The model under review builds one solid part; all positions refer to its coordinate system, in mm. Face numbers are marked on the shaded views. A direction names the side the tool comes from. Round coordinates to 2 decimals unless told otherwise and drop trailing zeros. Loops run counter-clockwise (first coordinate to the right, second up) from the corner with the lowest first, then second, coordinate; pieces in that order, holes last. Notation, with made-up numbers: M 34,-24.5 L 52,-24.5 A33 cw 52,9.5 Z; hole C 82.25,44 d8. An arc over 180 degrees is marked long. Answer in a Markdown table with one row per item. Add a question column.
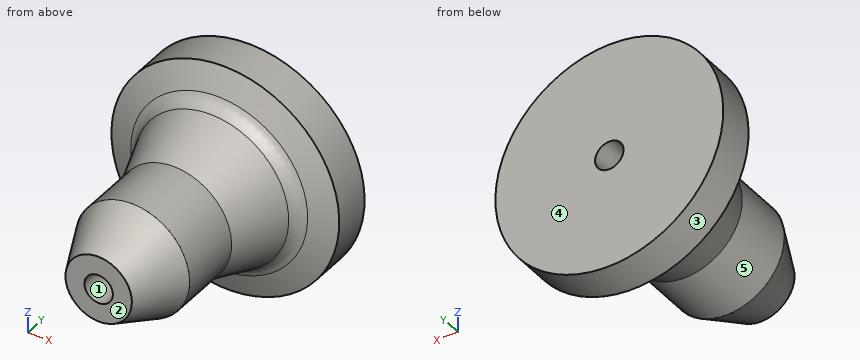
from build123d import *

# Parameters (mm, degrees)
F2_R = 10


with BuildPart() as f1:
    # F0 (on Right) → F1 (revolve)
    with BuildSketch(Plane.YZ):
        Polygon((0, 17.5), (0, 7.5), (120, 7.5), (120, 60), (100, 60), (93.521651, 42.200883), (60, 30), (26.806337, 30), align=None)
    revolve(axis=Axis((0, 51.72596, 0), (0, 1, 0)))

    # F2
    f2_edges = [f1.edges().sort_by_distance(p)[0] for p in [
        (0, 93.521651, -42.200883),
    ]]
    fillet(f2_edges, radius=F2_R)


solid = f1.part
1. Mouldability with a two-part tool opening along X and no side actions: class the marked faces 1, 2 and 3 as released by +X, released by -X, zero draft, split by the parting line, or undercut.
2. To check wall thickness, follow probe 1 along X at (y, z) = (33.5, 0); probe 2 along X at (y, z) = (94, 0); probe 3 along Z at (x, y) = (28, 103). State the ranges of each line that lie inside material, in increasing order.
3. Take a section at B-B, the plane y = 33.5. State the section outline as (x, z) points, and give its area (3 significant figures).
4. Take a section at A-A, the plane y = 66.5. State the section outline as (x, z) points.
5. Machinability: for the marked faces 4 and 5, which of the approach directions +Z, -Z, +X, -X, +Y, -Y give a long, thin tool a straight path to every point of the face, cutting with its end or side? Answer none if there is none.
6. For pin 1 Ø1 at (x, z) = (-29, 2) entering from -Y; pin 2 Ø2 at (x, y) = (4.5, 102) entering from +Z; pin 3 Ø3 at (y, z) = (45, 17) entering from -X, all flat-tipped, find the tip position at first contact; note any pin that passes through.
Check sheet entries:
| question | item | result |
|---|---|---|
| 1 | face 1 | undercut |
| 1 | face 2 | zero draft |
| 1 | face 3 | split by the parting line |
| 2 | probe 1 | x = -30 to -7.5, 7.5 to 30 |
| 2 | probe 2 | x = -44.4 to -7.5, 7.5 to 44.4 |
| 2 | probe 3 | z = -53.07 to 53.07 |
| 3 | outline | C 0,0 d60; hole C 0,0 d15 |
| 3 | area | 2,650 mm^2 |
| 4 | outline | C 0,0 d64.73; hole C 0,0 d15 |
| 5 | face 4 | +Z, -Z, +X, -X, +Y |
| 5 | face 5 | -Y |
| 6 | pin 1 | stops at y = 23.74 |
| 6 | pin 2 | stops at z = 59.9 |
| 6 | pin 3 | stops at x = -25.69 |
